For this review, take the finished solid that the model builds, in its own axes (mm). Coordinates: 2 decimals unless noted, no trailing zeros. Write each loop counter-clockwise with the first axis right and the second up, starting at its lowest first coordinate (ties: lowest second). Pieces come first, ordered by that corner, then holes. Notation, with made-up numbers: (48, 22.25) - (87, 22.25) arc R19 ccw to (87, 27.25) - close; hole circle Ø4 at (-31.5, -28). An arc over 180 degrees is marked (long way). Write each question's results on one line, items separated by ' | '.
Autodesk Inventor part; units mm, degrees
ref_plane "YZ Plane" through (0, 0, 0) normal (1, 0, 0) x (0, 1, 0)
ref_plane "XZ Plane" through (0, 0, 0) normal (0, 1, 0) x (-1, 0, 0)
ref_plane "XY Plane" through (0, 0, 0) normal (0, 0, 1) x (1, 0, 0)
sketch "Sketch" plane through (0, 0, 0) normal (0, 0, 1) x (1, 0, 0)
  line L0 (0, 0) -> (0, 2.6)
  line L1 (0, 2.6) -> (0.0065, 2.6)
  line L2 (0.0065, 2.6) -> (1.44, 1.5)
  line L3 (1.44, 1.5) -> (6.001, 1.5)
  line L4 (6.001, 1.5) -> (6.001, 2.6)
  line L5 (0, 0) -> (7.801, 0)
  arc A0 (7.801, 0) -> (6.001, 2.6) centre (5.0232, 0) ccw
  line L6 (-0.2879, 0) -> (1.7274, 0)
  line L7 (0, -0.2166) -> (0, 1.2997)
  dimension "d0" = 5.2
  dimension "d1" = 3
  dimension "d2" = 5.2
  dimension "d3" = 1.44
  dimension "d4" = 1.8
  dimension "d5" = 6.001
  dimension "d6" = 37.5
revolve "Body" add sketch "Sketch" angle 360 about axis through (0, 0, 0) along (1, 0, 0)
equation "\"d0\" = KOD"
equation "\"d1\" = NND1"
equation "\"d2\" = KOD1"
equation "\"d3\" = KOH"
equation "\"d4\" = KOH1"
equation "\"d6\" = 0.5 * SEWI"
equation "\"KLG\" = 6"
equation "\"NND1\" = 3"
equation "\"KOH\" = 1.44"
equation "\"KOD\" = 5.2"
equation "\"SEWI\" = 75deg"
equation "\"KOH1\" = 1.8"
equation "\"KOD1\" = 5.2"
equation "\"KLGMIN\" = 1.8"
equation "\"NND\" = 3"
equation "\"KLGMAX\" = 6"
properties part number "DIN 661 - A 3 x 10" material "Steel, Mild"
Q1. Take a section at A-A on x = 5.5. State the section outline as (y, z) points.
Results found:
outline: circle Ø3 at (0, 0)
Q2. Wall thickness on line 1 along X through (y, z) = (0.95, -1.7); line 2 along X through (y, z) = (-1.95, -1.5); line 3 along Z through (x, y) = (4, -0.05): over which ranges is each line inside the solid? List them lowest first. Write a range as from..to.
Results found:
line 1: 0..0.86, 6..7 | line 2: 0..0.19, 6..6.31 | line 3: -1.5..1.5
Q3. For pin 1 (1 mm diameter, centred on x = 3.5, z = 1, fed in from +Y); pin 2 (1 mm diameter, centred on x = 6.5, y = 1.5, fed in from +Z); pin 3 (1 mm diameter, centred on x = 4, y = -0.5, fed in from -Z), all flat-tipped, find the tip position at first contact; note any pin that passes through.
Results found:
pin 1: y = 1.41 | pin 2: z = 2.27 | pin 3: z = -1.5
Q4. Mouldability with a two-part tool opening along X and no side actions: class faces 1 (the face through (3.75, -1.5, 0.07)), 2 (the face through (6.001, 2, 0)), 3 (the face through (0, 0, 0)) as pulls with the +X half, pulls with the -X half, needs draft (parallel to the pull), parting line crosses it, or undercut.
Results found:
face 1: undercut | face 2: undercut | face 3: pulls with the -X half
